Here's how the part is built. I have some questions about the finished solid (model axes, mm). Face numbers are marked on the shaded views. Coordinates: 2 decimals unless noted, no trailing zeros. Write each loop counter-clockwise with the first axis right and the second up, starting at its lowest first coordinate (ties: lowest second). Pieces come first, ordered by that corner, then holes.
(1) Imagine slicing it at A-A, the plane x = 8. List the corners of the cut face in (y, z) for me (1 decimal).
(2) Imagine slicing it at C-C, the plane z = 8.5. List the corners of the cut face in (x, y) for me (1 decimal), plus the area to 3 significant figures.
(3) Thinking about a two-plate mould opening in X: for the marked faces 1, 2 and 3, which applies, released by +X, released by -X, zero draft, split by the parting line, or undercut?
(4) For pin 1 Ø4 at (x, z) = (17, -0.5) entering from -Y, with a flat end and sliding along its axis, tell me the tip position at first contact or that it passes through.
(5) Please list where these lines run through material, in increasing order: probe 1 along Z at (x, y) = (-5, -104.5); probe 2 along Z at (x, y) = (23.5, 293).
(6) Imagine slicing it at B-B, the plane y = -280. List the corners of the cut face in (x, z) for me.
```python
from build123d import *

# Parameters (mm, degrees)
F0_W     = 50.8
F0_H     = 50.8
F0_W_2   = 41.275
F0_H_2   = 41.275
F1_DEPTH = 403.225
F3_DEPTH = 50.8
F4_R     = 5.08


with BuildPart() as f1:
    # F0 (on Front) → F1 (new body, symmetric)
    with BuildSketch(Plane.XZ):
        Rectangle(F0_W, F0_H)
        Rectangle(F0_W_2, F0_H_2, mode=Mode.SUBTRACT)
    extrude(amount=F1_DEPTH, both=True)

    # F2 (on face) → F3 (cut)
    with BuildSketch(Plane(origin=(-25.4, 0, 0), x_dir=(0, -1, 0), z_dir=(-1, 0, 0))):
        Polygon((-352.425, 25.4), (-403.225, 25.4), (-403.225, -25.4), align=None)
    extrude(amount=-F3_DEPTH, mode=Mode.SUBTRACT)

    # F4
    f4_edges = [f1.edges().sort_by_distance(p)[0] for p in [
        (-25.4, -25.4, 25.4),
        (25.4, -25.4, 25.4),
        (20.6375, -2.38125, -20.6375),
        (-20.6375, -2.38125, -20.6375),
        (-25.4, 0, -25.4),
        (25.4, 0, -25.4),
    ]]
    fillet(f4_edges, radius=F4_R)


solid = f1.part
```
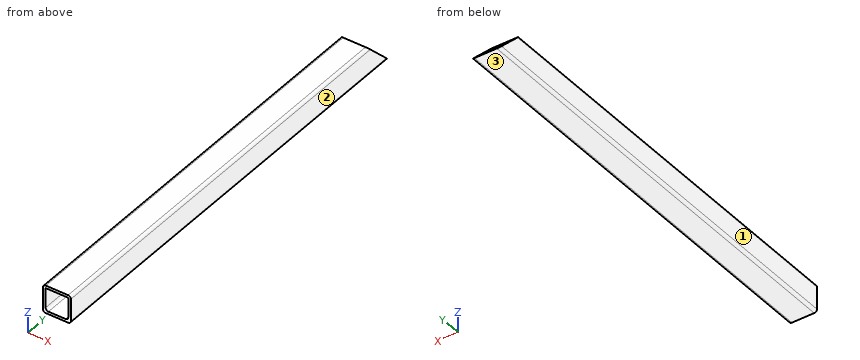
Recorded:
1. outline: (-403.2, -25.4) - (403.2, -25.4) - (398.5, -20.6) - (-403.2, -20.6) - close; (-403.2, 20.6) - (357.2, 20.6) - (352.4, 25.4) - (-403.2, 25.4) - close
2. outline: (-25.4, -403.2) - (-20.6, -403.2) - (-20.6, 369.3) - (-25.4, 369.3) - close; (20.6, -403.2) - (25.4, -403.2) - (25.4, 369.3) - (20.6, 369.3) - close
2. area: 7,360 mm2
3. face 1: released by -X
3. face 2: released by +X
3. face 3: zero draft
4. pin 1: passes through
5. probe 1: z = -25.4 to -20.64, 20.64 to 25.4
5. probe 2: z = -24.28 to 24.28
6. outline: (-25.4, -20.32) arc R5.08 ccw to (-20.32, -25.4) - (20.32, -25.4) arc R5.08 ccw to (25.4, -20.32) - (25.4, 20.32) arc R5.08 ccw to (20.32, 25.4) - (-20.32, 25.4) arc R5.08 ccw to (-25.4, 20.32) - close; hole (-20.64, -15.56) arc R5.08 ccw to (-15.56, -20.64) - (15.56, -20.64) arc R5.08 ccw to (20.64, -15.56) - (20.64, 20.64) - (-20.64, 20.64) - close
